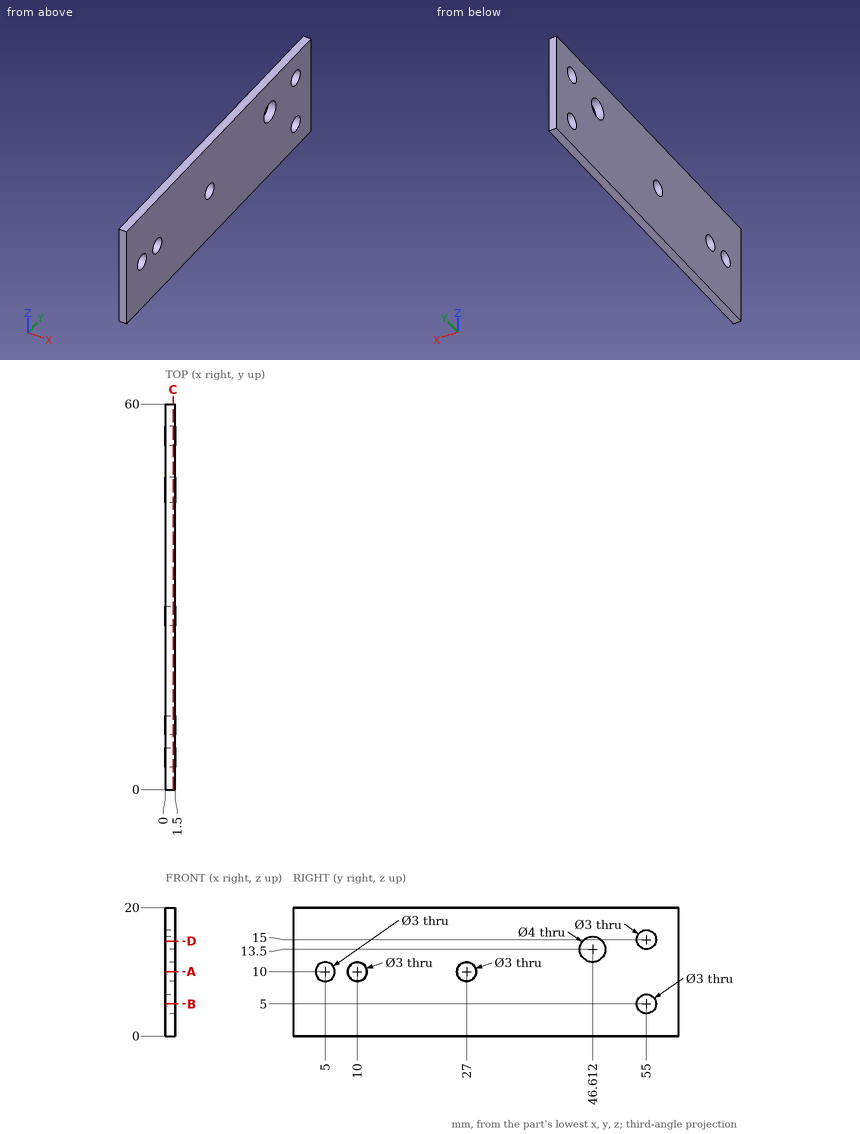
The figure shows three views and two pictorial views of one solid part (mm, origin at its lowest corner). Answer the questions. Coordinates: 2 decimals unless noted, no trailing zeros. Loops run counter-clockwise (first coordinate to the right, second up) from the corner with the lowest first, then second, coordinate; pieces in that order, holes last. Notation, with made-up numbers: (-29, 15.5) -> (16, 15.5) arc R23 cw to (16, 23.5) -> close; hole circle Ø8 at (-32, 0.5). An arc over 180 degrees is marked (long way). Return JSON: item names as keys, results as strings. Group by question number.
(1) Find the intervals of material crossed by probe 1 along Z at (x, y) = (1.05, 27); probe 2 along Y at (x, z) = (0.9, 5); probe 3 along Y at (x, z) = (1.25, 13.75), in increasing order. Write a range as from..to.
(2) A cutting plane is placed at B-B on z = 5. Write down the section's boundary in (x, y).
(3) Given pin 1 Ø1.8 at (y, z) = (55, 15) entering from -X, flat-ended and moving along its own axis, determine where the tip first touches the part or whether it passes through.
(4) A cutting plane is placed at A-A on z = 10. Write down the section's boundary in (x, y), and give its area (3 significant figures).
(5) A cutting plane is placed at D-D on z = 14.75. Write down the section's boundary in (x, y).
(6) A cutting plane is placed at C-C on x = 1.2. Write down the section's boundary in (y, z).
The answers:
{
 "1": {"probe 1": "z = 0..8.5, 11.5..20", "probe 2": "y = 0..53.5, 56.5..60", "probe 3": "y = 0..44.63, 48.6..54.17, 55.83..60"},
 "2": {"outline": "(0, 0) -> (1.5, 0) -> (1.5, 53.5) -> (0, 53.5) -> close; (0, 56.5) -> (1.5, 56.5) -> (1.5, 60) -> (0, 60) -> close"},
 "3": {"pin 1": "passes through"},
 "4": {"outline": "(0, 0) -> (1.5, 0) -> (1.5, 3.5) -> (0, 3.5) -> close; (0, 6.5) -> (1.5, 6.5) -> (1.5, 8.5) -> (0, 8.5) -> close; (0, 11.5) -> (1.5, 11.5) -> (1.5, 25.5) -> (0, 25.5) -> close; (0, 28.5) -> (1.5, 28.5) -> (1.5, 60) -> (0, 60) -> close", "area": "76.5 mm^2"},
 "5": {"outline": "(0, 0) -> (1.5, 0) -> (1.5, 45.05) -> (0, 45.05) -> close; (0, 48.17) -> (1.5, 48.17) -> (1.5, 53.52) -> (0, 53.52) -> close; (0, 56.48) -> (1.5, 56.48) -> (1.5, 60) -> (0, 60) -> close"},
 "6": {"outline": "(0, 0) -> (60, 0) -> (60, 20) -> (0, 20) -> close; hole circle Ø3 at (5, 10); hole circle Ø3 at (10, 10); hole circle Ø3 at (27, 10); hole circle Ø4 at (46.61, 13.5); hole circle Ø3 at (55, 5); hole circle Ø3 at (55, 15)"}
}
